For this review, take the finished solid that the model builds, in its own axes (mm). Coordinates: 2 decimals unless noted, no trailing zeros. Loops run counter-clockwise (first coordinate to the right, second up) from the corner with the lowest first, then second, coordinate; pieces in that order, holes last. Notation, with made-up numbers: (78.25, 3.25) - (105.25, 3.25) arc R14 cw to (105.25, 23.25) - close; hole circle Ø5 at (-0.75, 76). An arc over 180 degrees is marked (long way). Use one line per item in the form item = value. Start each with the question number.
1. To check wall thickness, follow probe 1 along X at (y, z) = (-1.8, -53); probe 2 along Z at (x, y) = (0, -1.1); probe 3 along Y at (x, z) = (8, -56.5). State the ranges of each line that lie inside material, in increasing order.
2. For pin 1 Ø1.5 at (y, z) = (-1.5, -12) entering from +X; pin 2 Ø3.5 at (y, z) = (-1.5, -197.5) entering from +X; pin 3 Ø2.5 at (y, z) = (-1, -171) entering from -X, all flat-tipped, find the tip position at first contact; note any pin that passes through.
3. Add section B-B on z = -59. Give the boundary of the cut face in (x, y), and give its area (3 significant figures).
4. Add section C-C on z = -137. Give the boundary of the cut face in (x, y), and give its area (3 significant figures).
5. Add section A-A on x = 0. Give the boundary of the cut face in (y, z), and give its area (3 significant figures).
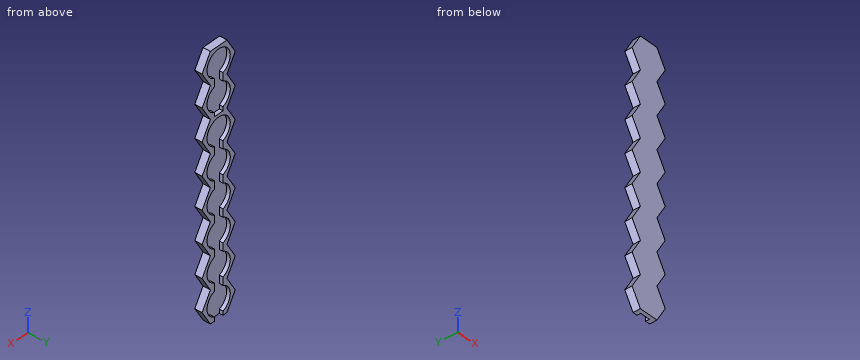
```python
from build123d import *

# Parameters (mm, degrees)
BOSS_EXTRUDE1_DEPTH = 6
SKETCH2_R           = 10.75
CUT_EXTRUDE1_DEPTH  = 3
SKETCH4_W           = 8
SKETCH4_H           = 3.271898978
CUT_EXTRUDE2_DEPTH  = 3
LPATTERN1_COUNT     = 2
LPATTERN1_PITCH     = 26.5
SKETCH6_W           = 8
SKETCH6_H           = 3
CUT_EXTRUDE3_DEPTH  = 32.182259914
LPATTERN2_START     = -6
LPATTERN2_DEPTH     = 3
LPATTERN2_START_2   = -3
LPATTERN2_2_DEPTH   = 3


# Read off the part's stored shape, not the designer's step: LPattern2
with BuildPart() as part:
    # Sketch3 → Boss-Extrude1 (new body)
    with BuildSketch(Plane(origin=(0, 0, 0), x_dir=(1, 0, 0), z_dir=(0, 1, 0))):
        Polygon((15.299782134, 0), (7.649891067, 13.25), (-7.649891067, 13.25), (-15.299782134, 0), (-7.649891067, -13.25), (7.649891067, -13.25), align=None)
    boss_extrude1 = extrude(amount=-BOSS_EXTRUDE1_DEPTH)

    # Sketch2 → Cut-Extrude1 (cut)
    with BuildSketch(Plane(origin=(0, 0, 0), x_dir=(1, 0, 0), z_dir=(0, 1, 0))):
        with Locations(Location((0, 0, 0), (0, 0, 270))):
            Circle(SKETCH2_R)
    cut_extrude1 = extrude(amount=-CUT_EXTRUDE1_DEPTH, mode=Mode.SUBTRACT)

    # Sketch4 → Cut-Extrude2 (cut)
    with BuildSketch(Plane(origin=(0, 0, 0), x_dir=(1, 0, 0), z_dir=(0, 1, 0))):
        with Locations((0, 11.614050511)):
            Rectangle(SKETCH4_W, SKETCH4_H)
    cut_extrude2 = extrude(amount=-CUT_EXTRUDE2_DEPTH, mode=Mode.SUBTRACT)

    # LPattern1: Boss-Extrude1, Cut-Extrude1, Cut-Extrude2 ×2
    with Locations(*[(0, 0, -i * LPATTERN1_PITCH) for i in range(1, LPATTERN1_COUNT)]):
        add(boss_extrude1)
        add(cut_extrude1, mode=Mode.SUBTRACT)
        add(cut_extrude2, mode=Mode.SUBTRACT)

    # Sketch6 → Cut-Extrude3 (cut, through all)
    with BuildSketch(Plane.XY.offset(-13.25)):
        with Locations((0, -1.5)):
            Rectangle(SKETCH6_W, SKETCH6_H)
    extrude(amount=-CUT_EXTRUDE3_DEPTH, mode=Mode.SUBTRACT)

    # LPattern2 outline → LPattern2 (add)
    with BuildSketch(Plane(origin=(0, 0, 0), x_dir=(1, 0, 0), z_dir=(0, 1, 0)).offset(LPATTERN2_START)):
        Polygon((-7.649891067, 198.75), (-15.299782134, 185.5), (-7.649891067, 172.25), (-15.299782134, 159), (-7.649891067, 145.75), (-15.299782134, 132.5), (-7.649891067, 119.25), (-15.299782134, 106), (-7.649891067, 92.75), (-15.299782134, 79.5), (-7.649891067, 66.25), (-15.299782134, 53), (-7.649891067, 39.75), (7.649891067, 39.75), (15.299782134, 53), (7.649891067, 66.25), (15.299782134, 79.5), (7.649891067, 92.75), (15.299782134, 106), (7.649891067, 119.25), (15.299782134, 132.5), (7.649891067, 145.75), (15.299782134, 159), (7.649891067, 172.25), (15.299782134, 185.5), (7.649891067, 198.75), align=None)
    extrude(amount=LPATTERN2_DEPTH)

    # LPattern2 2 outline → LPattern2 2 (add)
    with BuildSketch(Plane(origin=(0, 0, 0), x_dir=(1, 0, 0), z_dir=(0, 1, 0)).offset(LPATTERN2_START_2)):
        with BuildLine():
            ThreePointArc((-4, 69.521898978), (-10.75, 79.5), (-4, 89.478101022))
            Line((-4, 89.478101022), (-4, 96.021898978))
            ThreePointArc((-4, 96.021898978), (-10.75, 106), (-4, 115.978101022))
            Line((-4, 115.978101022), (-4, 122.521898978))
            ThreePointArc((-4, 122.521898978), (-10.75, 132.5), (-4, 142.478101022))
            Line((-4, 142.478101022), (-4, 149.021898978))
            ThreePointArc((-4, 149.021898978), (-10.75, 159), (-4, 168.978101022))
            Line((-4, 168.978101022), (-4, 175.521898978))
            ThreePointArc((-4, 175.521898978), (-10.75, 185.5), (-4, 195.478101022))
            Line((-4, 195.478101022), (-4, 198.75))
            Line((-4, 198.75), (-7.649891067, 198.75))
            Line((-7.649891067, 198.75), (-15.299782134, 185.5))
            Line((-15.299782134, 185.5), (-7.649891067, 172.25))
            Line((-7.649891067, 172.25), (-15.299782134, 159))
            Line((-15.299782134, 159), (-7.649891067, 145.75))
            Line((-7.649891067, 145.75), (-15.299782134, 132.5))
            Line((-15.299782134, 132.5), (-7.649891067, 119.25))
            Line((-7.649891067, 119.25), (-15.299782134, 106))
            Line((-15.299782134, 106), (-7.649891067, 92.75))
            Line((-7.649891067, 92.75), (-15.299782134, 79.5))
            Line((-15.299782134, 79.5), (-7.649891067, 66.25))
            Line((-7.649891067, 66.25), (-15.299782134, 53))
            Line((-15.299782134, 53), (-7.649891067, 39.75))
            Line((-7.649891067, 39.75), (7.649891067, 39.75))
            Line((7.649891067, 39.75), (15.299782134, 53))
            Line((15.299782134, 53), (7.649891067, 66.25))
            Line((7.649891067, 66.25), (15.299782134, 79.5))
            Line((15.299782134, 79.5), (7.649891067, 92.75))
            Line((7.649891067, 92.75), (15.299782134, 106))
            Line((15.299782134, 106), (7.649891067, 119.25))
            Line((7.649891067, 119.25), (15.299782134, 132.5))
            Line((15.299782134, 132.5), (7.649891067, 145.75))
            Line((7.649891067, 145.75), (15.299782134, 159))
            Line((15.299782134, 159), (7.649891067, 172.25))
            Line((7.649891067, 172.25), (15.299782134, 185.5))
            Line((15.299782134, 185.5), (7.649891067, 198.75))
            Line((7.649891067, 198.75), (4, 198.75))
            Line((4, 198.75), (4, 195.478101022))
            ThreePointArc((4, 195.478101022), (10.75, 185.5), (4, 175.521898978))
            Line((4, 175.521898978), (4, 168.978101022))
            ThreePointArc((4, 168.978101022), (10.75, 159), (4, 149.021898978))
            Line((4, 149.021898978), (4, 142.478101022))
            ThreePointArc((4, 142.478101022), (10.75, 132.5), (4, 122.521898978))
            Line((4, 122.521898978), (4, 115.978101022))
            ThreePointArc((4, 115.978101022), (10.75, 106), (4, 96.021898978))
            Line((4, 96.021898978), (4, 89.478101022))
            ThreePointArc((4, 89.478101022), (10.75, 79.5), (4, 69.521898978))
            Line((4, 69.521898978), (4, 62.978101022))
            ThreePointArc((4, 62.978101022), (0, 42.25), (-4, 62.978101022))
            Line((-4, 62.978101022), (-4, 69.521898978))
        make_face()
    extrude(amount=LPATTERN2_2_DEPTH)


solid = part.part
```
Conclusion:
q1.probe_1 = -15.3 to -10.75, 10.75 to 15.3
q1.probe_2 = -42.25 to -39.75, 10.75 to 13.25
q1.probe_3 = -6 to -3
q2.pin_1 = 8.8
q2.pin_2 = 9.38
q2.pin_3 = -9.09
q3.outline = (-11.84, -6) - (11.84, -6) - (11.84, 0) - (8.92, 0) - (8.92, -3) - (-8.92, -3) - (-8.92, 0) - (-11.84, 0) - close
q3.area = 88.5 mm^2
q4.outline = (-12.7, -6) - (12.7, -6) - (12.7, 0) - (9.76, 0) - (9.76, -3) - (-9.76, -3) - (-9.76, 0) - (-12.7, 0) - close
q4.area = 93.8 mm^2
q5.outline = (-6, -198.75) - (-3, -198.75) - (-3, -42.25) - (0, -42.25) - (0, -39.75) - (-3, -39.75) - (-3, 10.75) - (0, 10.75) - (0, 13.25) - (-6, 13.25) - close
q5.area = 651 mm^2
